```python
from build123d import *

# Parameters (mm, degrees)
F2_DEPTH      = 2.54
F3_DEPTH      = 7.62
F5_DEPTH      = 12.7
F7_ANGLE      = 15
F8_T2_ANGLE   = 20.2683164311
F8_T4_ANGLE   = 18.6436758241
F10_ANGLE     = 15
F11_T2_ANGLE  = 15
F11_T4_ANGLE  = 15
F11_T5_DEPTH  = 18.5785787418
F11_T7_DEPTH  = 18.5785787418
F11_T10_ANGLE = 17.3026091046
F11_T12_ANGLE = 17.3227523422
F11_T14_ANGLE = 17.3991627069
F11_T16_ANGLE = 17.6093282682


# Not quite as in the source:
# - a fillet or chamfer that OpenCascade refuses, or shapes differently, is made with other operations: its cross-section is extruded or revolved along the edge and cut away or added


with BuildPart() as f2:
    # F1 (on Top) → F2 (new body)
    with BuildSketch(Plane.XY):
        with BuildLine():
            ThreePointArc((36.1159330774, -134.7864972077), (18.2137880201, -138.3474552622), (0, -139.54125))
            Line((0, -139.54125), (0, -142.08125))
            ThreePointArc((0, -142.08125), (18.5453245484, -140.8657252101), (36.773333452, -137.2399488064))
            Line((36.773333452, -137.2399488064), (36.1159330774, -134.7864972077))
        make_face()
        with BuildLine():
            ThreePointArc((36.773333452, -137.2399488064), (18.5453245484, -140.8657252101), (0, -142.08125))
            Line((0, -142.08125), (0, -149.225))
            ThreePointArc((0, -149.225), (19.477771034, -147.9483594385), (38.6222720054, -144.140281428))
            Line((38.6222720054, -144.140281428), (36.773333452, -137.2399488064))
        make_face()
        with BuildLine():
            ThreePointArc((38.6222720054, -144.140281428), (19.477771034, -147.9483594385), (0, -149.225))
            Line((0, -149.225), (0, -151.765))
            ThreePointArc((0, -151.765), (19.8093075623, -150.4666293864), (39.27967238, -146.5937330268))
            Line((39.27967238, -146.5937330268), (38.6222720054, -144.140281428))
        make_face()
    extrude(amount=F2_DEPTH)

    # F1 (on Top) → F3 (join)
    with BuildSketch(Plane.XY):
        with BuildLine():
            ThreePointArc((36.1159330774, -134.7864972077), (18.2137880201, -138.3474552622), (0, -139.54125))
            Line((0, -139.54125), (0, -142.08125))
            ThreePointArc((0, -142.08125), (18.5453245484, -140.8657252101), (36.773333452, -137.2399488064))
            Line((36.773333452, -137.2399488064), (36.1159330774, -134.7864972077))
        make_face()
    extrude(amount=-F3_DEPTH)

    # F4 (on face) → F5 (join)
    with BuildSketch(Plane.XY):
        with BuildLine():
            ThreePointArc((38.6880120429, -144.3856265879), (19.5109246869, -148.2001864333), (0, -149.479))
            Line((0, -149.479), (0, -151.765))
            ThreePointArc((0, -151.765), (19.8093075623, -150.4666293864), (39.27967238, -146.5937330268))
            Line((39.27967238, -146.5937330268), (38.6880120429, -144.3856265879))
        make_face()
    extrude(amount=-F5_DEPTH)

    # F6 (on face) → F7 (revolve)
    with BuildSketch(Plane(origin=(0, 0, 0), x_dir=(0, -1, 0), z_dir=(-1, 0, 0))):
        Polygon((147.574, -7.112), (149.479, -12.7), (149.479, -7.112), align=None)
    revolve(axis=Axis((0, 0, 0), (0, 0, 1)), revolution_arc=F7_ANGLE)

    # F8: chamfer of 2.54 on 2 edges, made by hand

    # F8_s1 → F8_t2 (revolve, cut)
    with BuildSketch(Plane(origin=(0, 0, 0), x_dir=(0, 0, 1), z_dir=(-0.9989433481, 0.0459585396, 0))):
        Polygon((-7.62, -139.54125), (-5.08, -142.08125), (-7.62, -142.08125), align=None)
    revolve(axis=Axis((0, 0, -7.62), (0, 0, 1)), revolution_arc=F8_T2_ANGLE, mode=Mode.SUBTRACT)

    # F8_s3 → F8_t4 (revolve, cut)
    with BuildSketch(Plane(origin=(0, 0, 0), x_dir=(0, 0, 1), z_dir=(0.9572092654, 0.289396652, 0))):
        Polygon((-12.7, 151.2966330745), (-10.9795917766, 148.8924971966), (-12.7, 149.479), align=None)
    revolve(axis=Axis((0, 0, -12.7), (0, 0, -1)), revolution_arc=F8_T4_ANGLE, mode=Mode.SUBTRACT)

    # F9 (on face) → F10 (revolve)
    with BuildSketch(Plane(origin=(0, 0, 0), x_dir=(0, -1, 0), z_dir=(-1, 0, 0))):
        Polygon((158.1288493504, -9.8370487633), (151.765, -5.7552899175), (151.765, -8.7728602812), (156.7575335503, -11.9750602171), align=None)
        Polygon((151.765, -8.7728602812), (151.765, -5.7552899175), (151.765, 2.54), (139.54125, 2.54), (139.54125, -7.62), (142.08125, -5.08), (142.08125, 0), (149.479, 0), (149.479, -7.112), (147.574, -7.112), (148.8924971966, -10.9795917766), (151.2966330745, -12.7), (151.765, -12.7), align=None)
    revolve(axis=Axis((0, 0, 0), (0, 0, 1)), revolution_arc=F10_ANGLE)

    # F11: fillet of radius 1.27 on 8 edges, made by hand

    # F11_s1 → F11_t2 (revolve)
    with BuildSketch(Plane.YZ):
        with BuildLine():
            ThreePointArc((-151.7646, -5.0599866722), (-151.9205140931, -5.6702824854), (-152.3500463685, -6.1310125674))
            Line((-152.3500463685, -6.1310125674), (-152.2813510053, -6.2381151569))
            ThreePointArc((-152.2813510053, -6.2381151569), (-151.9889357987, -6.0500854846), (-151.6963046368, -5.862392507))
            Line((-151.6963046368, -5.862392507), (-151.63776, -5.7552899175))
            ThreePointArc((-151.63776, -5.7552899175), (-151.63776, -5.4076382949), (-151.63736, -5.0599866722))
            Line((-151.63736, -5.0599866722), (-151.7646, -5.0599866722))
        make_face()
    revolve(axis=Axis((0, 0, -5.7552899175), (0, 0, 1)), revolution_arc=F11_T2_ANGLE)

    # F11_s3 → F11_t4 (revolve)
    with BuildSketch(Plane.YZ):
        with BuildLine():
            ThreePointArc((-151.7646, -11.0968951513), (-152.4258553263, -9.9818406517), (-153.7214416132, -10.0272423808))
            Line((-153.7214416132, -10.0272423808), (-153.7900489045, -9.9202771037))
            ThreePointArc((-153.7900489045, -9.9202771037), (-152.8117201202, -9.2932544013), (-151.8336072912, -8.6658950041))
            Line((-151.8336072912, -8.6658950041), (-151.6379231299, -8.7728602812))
            ThreePointArc((-151.6379231299, -8.7728602812), (-151.6379231299, -9.9348777163), (-151.6375231299, -11.0968951513))
            Line((-151.6375231299, -11.0968951513), (-151.7646, -11.0968951513))
        make_face()
    revolve(axis=Axis((0, 0, -8.7728602812), (0, 0, 1)), revolution_arc=F11_T4_ANGLE)

    # F11_s6 → F11_t5 (cut)
    with BuildSketch(Plane.XZ.offset(136.3638356291)):
        with BuildLine():
            ThreePointArc((1.2709656854, 2.5404), (0.3719743879, 2.1680256121), (-0.0004, 1.2690343146))
            Line((-0.0004, 1.2690343146), (-0.1275365685, 1.2690343146))
            ThreePointArc((-0.1275365685, 1.2690343146), (-0.1271365685, 1.9045171573), (-0.1271365685, 2.54))
            Line((-0.1271365685, 2.54), (0, 2.6671365685))
            ThreePointArc((0, 2.6671365685), (0.6354828427, 2.6671365685), (1.2709656854, 2.6675365685))
            Line((1.2709656854, 2.6675365685), (1.2709656854, 2.5404))
        make_face()
    extrude(amount=F11_T5_DEPTH, mode=Mode.SUBTRACT)

    # F11_s8 → F11_t7 (cut)
    with BuildSketch(Plane(origin=(40.1020477334, -149.6628796285, 0), x_dir=(0, 0, 1), z_dir=(-0.2588190451, 0.9659258263, 0))):
        with BuildLine():
            ThreePointArc((1.2690343146, 0.0004), (2.1680256121, -0.3719743879), (2.5404, -1.2709656854))
            Line((2.5404, -1.2709656854), (2.6675365685, -1.2709656854))
            ThreePointArc((2.6675365685, -1.2709656854), (2.6671365685, -0.6354828427), (2.6671365685, 0))
            Line((2.6671365685, 0), (2.54, 0.1271365685))
            ThreePointArc((2.54, 0.1271365685), (1.9045171573, 0.1271365685), (1.2690343146, 0.1275365685))
            Line((1.2690343146, 0.1275365685), (1.2690343146, 0.0004))
        make_face()
    extrude(amount=F11_T7_DEPTH, mode=Mode.SUBTRACT)

    # F11_s9 → F11_t10 (revolve, cut)
    with BuildSketch(Plane(origin=(0, 0, 0), x_dir=(0, 0, 1), z_dir=(-0.9997981213, 0.0200927029, 0))):
        with BuildLine():
            ThreePointArc((-9.1505328065, -157.0592467258), (-9.9493287423, -157.6149202728), (-10.9070832984, -157.443006783))
            Line((-10.9070832984, -157.443006783), (-10.9757228201, -157.5500223104))
            ThreePointArc((-10.9757228201, -157.5500223104), (-10.440597575, -157.8927752468), (-9.9056882851, -158.2358648778))
            Line((-9.9056882851, -158.2358648778), (-9.7300332359, -158.1974888721))
            ThreePointArc((-9.7300332359, -158.1974888721), (-9.3869436048, -157.6625795822), (-9.043517279, -157.1278862476))
            Line((-9.043517279, -157.1278862476), (-9.1505328065, -157.0592467258))
        make_face()
    revolve(axis=Axis((0, 0, -9.8370487633), (0, 0, 1)), revolution_arc=F11_T10_ANGLE, mode=Mode.SUBTRACT)

    # F11_s11 → F11_t12 (revolve, cut)
    with BuildSketch(Plane(origin=(0, 0, 0), x_dir=(0, 0, 1), z_dir=(-0.9997945739, 0.02026845, 0))):
        with BuildLine():
            ThreePointArc((-10.9054575925, -157.4440495071), (-11.4611311395, -156.6452535713), (-11.2892176497, -155.6874990152))
            Line((-11.2892176497, -155.6874990152), (-11.3962331771, -155.6188594935))
            ThreePointArc((-11.3962331771, -155.6188594935), (-11.7389861135, -156.1539847386), (-12.0820757445, -156.6888940285))
            Line((-12.0820757445, -156.6888940285), (-12.0436997388, -156.8645490777))
            ThreePointArc((-12.0436997388, -156.8645490777), (-11.5087904489, -157.2076387088), (-10.9740971142, -157.5510650346))
            Line((-10.9740971142, -157.5510650346), (-10.9054575925, -157.4440495071))
        make_face()
    revolve(axis=Axis((0, 0, -11.9750602171), (0, 0, 1)), revolution_arc=F11_T12_ANGLE, mode=Mode.SUBTRACT)

    # F11_s13 → F11_t14 (revolve, cut)
    with BuildSketch(Plane(origin=(0, 0, 0), x_dir=(0, 0, 1), z_dir=(-0.9997808365, 0.0209351147, 0))):
        with BuildLine():
            ThreePointArc((2.5404, -150.4940343146), (2.1680256121, -151.3930256121), (1.2690343146, -151.7654))
            Line((1.2690343146, -151.7654), (1.2690343146, -151.8925365685))
            ThreePointArc((1.2690343146, -151.8925365685), (1.9045171573, -151.8921365685), (2.54, -151.8921365685))
            Line((2.54, -151.8921365685), (2.6671365685, -151.765))
            ThreePointArc((2.6671365685, -151.765), (2.6671365685, -151.1295171573), (2.6675365685, -150.4940343146))
            Line((2.6675365685, -150.4940343146), (2.5404, -150.4940343146))
        make_face()
    revolve(axis=Axis((0, 0, 2.54), (0, 0, 1)), revolution_arc=F11_T14_ANGLE, mode=Mode.SUBTRACT)

    # F11_s15 → F11_t16 (revolve, cut)
    with BuildSketch(Plane(origin=(0, 0, 0), x_dir=(0, 0, 1), z_dir=(0.9597824413, 0.2807448405, 0))):
        with BuildLine():
            ThreePointArc((1.2690343146, 139.54085), (2.1680256121, 139.9132243879), (2.5404, 140.8122156854))
            Line((2.5404, 140.8122156854), (2.6675365685, 140.8122156854))
            ThreePointArc((2.6675365685, 140.8122156854), (2.6671365685, 140.1767328427), (2.6671365685, 139.54125))
            Line((2.6671365685, 139.54125), (2.54, 139.4141134315))
            ThreePointArc((2.54, 139.4141134315), (1.9045171573, 139.4141134315), (1.2690343146, 139.4137134315))
            Line((1.2690343146, 139.4137134315), (1.2690343146, 139.54085))
        make_face()
    revolve(axis=Axis((0, 0, 2.54), (0, 0, -1)), revolution_arc=F11_T16_ANGLE, mode=Mode.SUBTRACT)


solid = f2.part
```
The model under review builds one solid part; all positions refer to its coordinate system, in mm. A direction names the side the tool comes from. Coordinates: 2 decimals unless noted, no trailing zeros. Order: outer loops, then holes, each group sorted by start corner. A loop starts at its lowest first (then second) coordinate and runs counter-clockwise, first axis right, second up. Notation, with made-up numbers: (16.5, 69) -> (58.5, 69) arc R21 cw to (58.5, 96) -> close; hole circle Ø5 at (3, 28). An arc over 180 degrees is marked (long way). Answer in a Markdown table with one row per item. Add a question column.
Item 1: We need section A-A on z = -3.5. Write out the cut boundary in (x, y) (1 decimal).
Item 2: Machinability: for faces 5 (the flat face through (19, -145, 0)), 6 (the cylindrical face through (18.29, -140.9, -2.5)), 7 (the cylindrical face through (19.782, -148.164, -3.506)), which of the approach directions +Z, -Z, +X, -X, +Y, -Y give a long, thin tool a straight path to every point of the face, cutting with its end or side? Answer none if there is none.
Item 3: We need section B-B on z = 1.75. Write out the cut boundary in (x, y).
Item 4: Mouldability with a two-part tool opening along Y and no side actions: class faces 1 (the conical face through (19.826, -148.493, -11.637)), 2 (the flat face through (19.5, -150.2, -12.7)), 3 (the conical face through (18, -139, -7)), 4 (the cylindrical face through (19.534, -150.503, -11.871)) as +Y half, -Y half, draft (parallel to the pull), parting line (faces both ways), or undercut.
Item 5: To check wall thickness, follow probe 1 along Y at (x, z) = (31, -10); probe 2 along Y at (x, z) = (12, -6.75); probe 3 along Z at (x, y) = (30, -148.25). State the ranges of each line that lie inside material, in increasing order.
Item 6: Clearance check with flat-ended pins moving along their axes: pin 1 (6 mm diameter, centred on x = 13, y = -146, fed in from -Z); pin 2 (6 mm diameter, centred on y = -140, z = -7.5, fed in from +X); pin 3 (1 mm diameter, centred on x = 30, z = -11, fed in from -Y). State where each tip first meets the part, or that it passes through.
Final values:
| question | item | result |
|---|---|---|
| 1 | outline | (0, -151.8) arc R151.8 ccw to (39.3, -146.6) -> (38.7, -144.4) arc R149.5 cw to (0, -149.5) -> close; (0, -142.1) arc R142.1 ccw to (36.8, -137.2) -> (36.1, -134.8) arc R139.5 cw to (0, -139.5) -> close |
| 2 | face 5 | none |
| 2 | face 6 | -Z, +X |
| 2 | face 7 | -X |
| 3 | outline | (0.09, -151.67) arc R151.67 ccw to (39.16, -146.53) -> (36.05, -134.9) arc R139.64 cw to (0.09, -139.64) -> close |
| 4 | face 1 | +Y half |
| 4 | face 2 | draft |
| 4 | face 3 | undercut |
| 4 | face 4 | undercut |
| 5 | probe 1 | y = -154.55 to -150.52, -149.21 to -145.29 |
| 5 | probe 2 | y = -152.85 to -149, -139.9 to -139.02 |
| 5 | probe 3 | z = -12.67 to 2.29 |
| 6 | pin 1 | stops at z = -11.47 |
| 6 | pin 2 | stops at x = 38.32 |
| 6 | pin 3 | stops at y = -154.76 |
